from build123d import *

# Parameters (mm, degrees)
SKETCH_1_R      = 2
EXTRUDE_1_DEPTH = 2.7


with BuildPart() as part:
    # 草图1 → 凸台-拉伸1 (new body)
    with BuildSketch(Plane.XY):
        with BuildLine():
            ThreePointArc((3, 25), (0.878679656, 24.121320344), (0, 22))
            Line((0, 22), (0, -22))
            ThreePointArc((0, -22), (0.878679656, -24.121320344), (3, -25))
            Line((3, -25), (247, -25))
            ThreePointArc((247, -25), (249.121320344, -24.121320344), (250, -22))
            Line((250, -22), (250, 22))
            ThreePointArc((250, 22), (249.121320344, 24.121320344), (247, 25))
            Line((247, 25), (3, 25))
        make_face()
        with Locations(Location((5, -13.35, 0), (0, 0, 180))):
            Circle(SKETCH_1_R, mode=Mode.SUBTRACT)
        with BuildLine():
            Line((184.15863574, -23.5), (64.15863574, -23.5))
            ThreePointArc((64.15863574, -23.5), (61.65863574, -21), (64.15863574, -18.5))
            Line((64.15863574, -18.5), (184.15863574, -18.5))
            ThreePointArc((184.15863574, -18.5), (185.926402692, -19.232233047), (186.65863574, -21))
            ThreePointArc((186.65863574, -21), (185.926402692, -22.767766953), (184.15863574, -23.5))
        make_face(mode=Mode.SUBTRACT)
        with BuildLine():
            ThreePointArc((185, -2.5), (182.5, 0), (185, 2.5))
            Line((185, 2.5), (235, 2.5))
            ThreePointArc((235, 2.5), (236.767766953, 1.767766953), (237.5, 0))
            ThreePointArc((237.5, 0), (236.767766953, -1.767766953), (235, -2.5))
            Line((235, -2.5), (185, -2.5))
        make_face(mode=Mode.SUBTRACT)
        with Locations(Location((5, 20.65, 0), (0, 0, 180))):
            Circle(SKETCH_1_R, mode=Mode.SUBTRACT)
        with Locations(Location((39, 20.65, 0), (0, 0, 180))):
            Circle(SKETCH_1_R, mode=Mode.SUBTRACT)
        with BuildLine():
            Line((184.15863574, 18.5), (64.15863574, 18.5))
            ThreePointArc((64.15863574, 18.5), (61.65863574, 21), (64.15863574, 23.5))
            Line((64.15863574, 23.5), (184.15863574, 23.5))
            ThreePointArc((184.15863574, 23.5), (185.926402692, 22.767766953), (186.65863574, 21))
            ThreePointArc((186.65863574, 21), (185.926402692, 19.232233047), (184.15863574, 18.5))
        make_face(mode=Mode.SUBTRACT)
    extrude(amount=EXTRUDE_1_DEPTH)


solid = part.part
Geometry check sheet. Reference: the model listing, model coordinates, mm. Round coordinates to 2 decimals unless told otherwise and drop trailing zeros. Loops run counter-clockwise (first coordinate to the right, second up) from the corner with the lowest first, then second, coordinate; pieces in that order, holes last.
Item 1: Cross-section at A-A on z = 1.2. Record the boundary of the cut face in (x, y), then the cut area to 3 significant figures.
Item 2: Gauge pin test, flat end, axial feed: pin 1 (3 mm diameter, centred on x = 169.5, y = 3, fed in from -Z). Record the tip position at first contact, or that the pin passes through.
Item 3: Mould release check, pull along X, two halves, no side actions. Record for faces 1 (the cylindrical face through (5.434, 22.602, 1.331)), 2 (the flat face through (123, 0, 2.7)): pulls with the +X half, pulls with the -X half, needs draft (parallel to the pull), parting line crosses it, or undercut.
Item 4: Cross-section at B-B on x = 118.5. Record the boundary of the cut face in (y, z).
Item 5: Thickness scan on line 1 (Y direction, x = 64.5, z = 0.8); line 2 (Y direction, x = 5, z = 2); line 3 (X direction, y = 20.65, z = 1.7). Record the ranges inside material, lowest first.
Answer sheet:
1. outline: (0, -22) arc R3 ccw to (3, -25) - (247, -25) arc R3 ccw to (250, -22) - (250, 22) arc R3 ccw to (247, 25) - (3, 25) arc R3 ccw to (0, 22) - close; hole circle Ø4 at (5, -13.35); hole circle Ø4 at (5, 20.65); hole circle Ø4 at (39, 20.65); hole (64.16, -23.5) - (184.16, -23.5) arc R2.5 ccw to (184.16, -18.5) - (64.16, -18.5) arc R2.5 ccw to start; hole (64.16, 18.5) - (184.16, 18.5) arc R2.5 ccw to (184.16, 23.5) - (64.16, 23.5) arc R2.5 ccw to start; hole (185, -2.5) - (235, -2.5) arc R2.5 ccw to (235, 2.5) - (185, 2.5) arc R2.5 ccw to start
1. area: 10,900 mm2
2. pin 1: stops at z = 0
3. face 1: undercut
3. face 2: needs draft
4. outline: (-25, 0) - (-23.5, 0) - (-23.5, 2.7) - (-25, 2.7) - close; (-18.5, 0) - (18.5, 0) - (18.5, 2.7) - (-18.5, 2.7) - close; (23.5, 0) - (25, 0) - (25, 2.7) - (23.5, 2.7) - close
5. line 1: y = -25 to -23.5, -18.5 to 18.5, 23.5 to 25
5. line 2: y = -25 to -15.35, -11.35 to 18.65, 22.65 to 25
5. line 3: x = 0 to 3, 7 to 37, 41 to 61.68, 186.63 to 250
